Could you check a few things on this model? Use its own coordinates, in mm. A direction names the side the tool comes from. Coordinates: 2 decimals unless noted, no trailing zeros. Loops run counter-clockwise (first coordinate to the right, second up) from the corner with the lowest first, then second, coordinate; pieces in that order, holes last.
1) For faces 4 (the face through (-62.5, -4, 0)), 5 (the face through (87.5, -4, 0)), which set-ups out of +Z, -Z, +X, -X, +Y, -Y let a thin tool reach every point of the face, with its end or its side?
2) Thinking about a two-plate mould opening in Z: for faces 1 (the face through (-71.284, -3.803, 29.385)), 2 (the face through (-87.5, -4, 0)), 3 (the face through (86, -3.8, 35.07)), which applies, released by +Z, released by -Z, zero draft, split by the parting line, or undercut?
3) Imagine slicing it at C-C on x = -46. Please give me the cut outline in (y, z).
4) If I drill on line 1 along Z through (x, y) = (-72.5, -5.5); line 2 along Z through (x, y) = (-47.5, -6.75); line 3 along X through (y, z) = (-5.75, 13), over which ranges is the centre line in solid material (lowest first)?
5) Imagine slicing it at B-B on z = 7.5. Please give me the cut outline in (x, y).
6) Imagine slicing it at A-A on x = 72.5. Please give me the cut outline in (y, z), plus the area to 3 significant figures.
7) Will this pin go through, and if not, where does the flat tip stop? P1, Ø5.5, axis at x = -72.5, z = -19, coming from the +Y side.
```python
from build123d import *

# Parameters (mm, degrees)
F0_W     = 175
F0_H     = 73
F0_W_2   = 99
F0_H_2   = 41
F1_DEPTH = 7.5
F2_R     = 5
F3_D     = 3.3


with BuildPart() as f1:
    # F0 (on Front) → F1 (new body)
    with BuildSketch(Plane.XZ):
        Rectangle(F0_W, F0_H)
        with Locations((-13, 0)):
            Rectangle(F0_W_2, F0_H_2, mode=Mode.SUBTRACT)
    extrude(amount=F1_DEPTH)

    # F2
    f2_edges = [f1.edges().sort_by_distance(p)[0] for p in [
        (-87.5, -3.75, 36.5),
        (87.5, -3.75, 36.5),
        (87.5, -3.75, -36.5),
        (-87.5, -3.75, -36.5),
    ]]
    fillet(f2_edges, radius=F2_R)

    # F3 (through all)
    with Locations(Plane(origin=(0, 0, 0), x_dir=(1, 0, 0), z_dir=(0, 1, 0))):
        with Locations((-72.5, -30.5), (-72.5, 19), (72.5, 19), (72.5, -30.5)):
            Hole(F3_D / 2)


solid = f1.part
```
Filled in:
1. face 4: +Y, -Y
1. face 5: +Z, -Z, +X, +Y, -Y
2. face 1: undercut
2. face 2: zero draft
2. face 3: released by +Z
3. outline: (-7.5, -36.5) - (0, -36.5) - (0, -20.5) - (-7.5, -20.5) - close; (-7.5, 20.5) - (0, 20.5) - (0, 36.5) - (-7.5, 36.5) - close
4. line 1: z = -36.5 to -20.65, -17.35 to 28.85, 32.15 to 36.5
4. line 2: z = -36.5 to -20.5, 20.5 to 36.5
4. line 3: x = -87.5 to -62.5, 36.5 to 87.5
5. outline: (-87.5, -7.5) - (-62.5, -7.5) - (-62.5, 0) - (-87.5, 0) - close; (36.5, -7.5) - (87.5, -7.5) - (87.5, 0) - (36.5, 0) - close
6. outline: (-7.5, -36.5) - (0, -36.5) - (0, -20.65) - (-7.5, -20.65) - close; (-7.5, -17.35) - (0, -17.35) - (0, 28.85) - (-7.5, 28.85) - close; (-7.5, 32.15) - (0, 32.15) - (0, 36.5) - (-7.5, 36.5) - close
6. area: 498 mm2
7. P1: stops at y = 0
